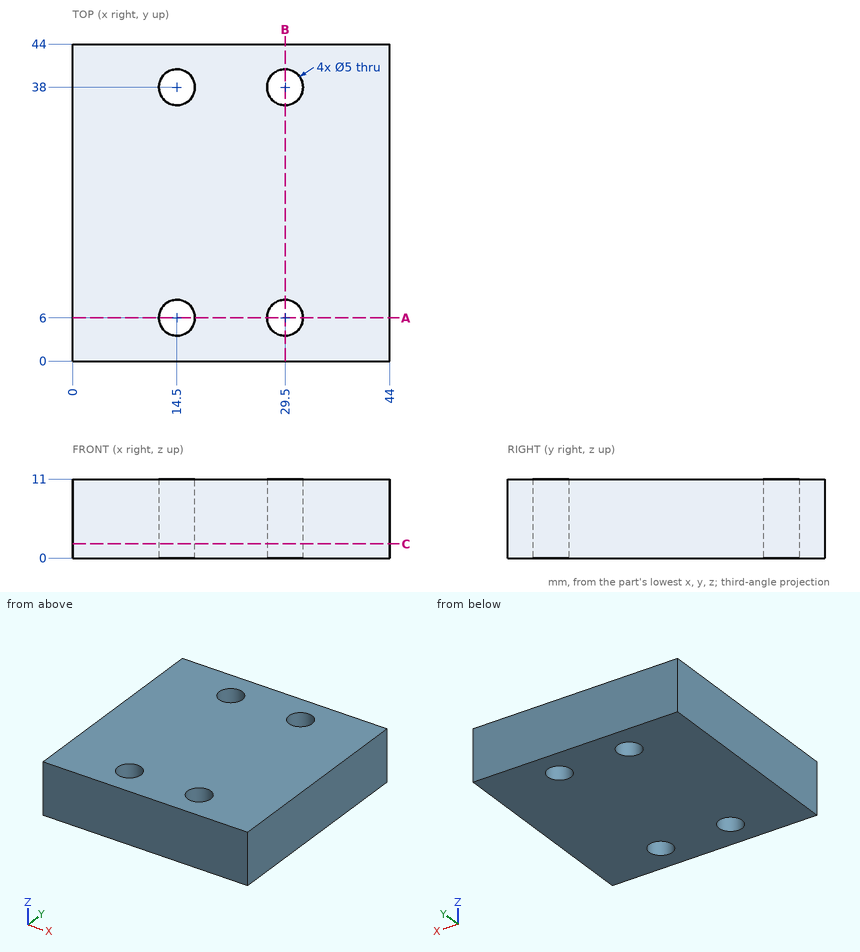
Drawing for the job (mm, zero at the part's lowest x, y, z). Round coordinates to 2 decimals unless told otherwise and drop trailing zeros. Loops run counter-clockwise (first coordinate to the right, second up) from the corner with the lowest first, then second, coordinate; pieces in that order, holes last.
1. Drop a flat-ended pin along its axis: P1, Ø4, axis at x = 14.5, y = 6, coming from the +Z side. Give the stop position or say it passes through.
Check values:
P1: passes through
2. Band-saw the part on B-B, the plane x = 29.5. List the corners of the cut face in (y, z), and give its area (3 significant figures).
Check values:
outline: (0, 0) - (3.5, 0) - (3.5, 11) - (0, 11) - close; (8.5, 0) - (35.5, 0) - (35.5, 11) - (8.5, 11) - close; (40.5, 0) - (44, 0) - (44, 11) - (40.5, 11) - close
area: 374 mm2
3. Wall check: probe 1 along Y at (x, z) = (14.5, 7.25); probe 2 along X at (y, z) = (6, 6); probe 3 along Y at (x, z) = (27.5, 3.5). Give the ranges that are in metal, low to high.
Check values:
probe 1: y = 0 to 3.5, 8.5 to 35.5, 40.5 to 44
probe 2: x = 0 to 12, 17 to 27, 32 to 44
probe 3: y = 0 to 4.5, 7.5 to 36.5, 39.5 to 44
4. Band-saw the part on A-A, the plane y = 6. List the corners of the cut face in (x, z), and give its area (3 significant figures).
Check values:
outline: (0, 0) - (12, 0) - (12, 11) - (0, 11) - close; (17, 0) - (27, 0) - (27, 11) - (17, 11) - close; (32, 0) - (44, 0) - (44, 11) - (32, 11) - close
area: 374 mm2
5. Band-saw the part on C-C, the plane z = 2. List the corners of the cut face in (x, y).
Check values:
outline: (0, 0) - (44, 0) - (44, 44) - (0, 44) - close; hole circle Ø5 at (14.5, 6); hole circle Ø5 at (14.5, 38); hole circle Ø5 at (29.5, 6); hole circle Ø5 at (29.5, 38)
